```python
from build123d import *

# Parameters (mm, degrees)
F0_W     = 30.4
F0_H     = 20.2
F1_DEPTH = 16
F0_W_2   = 32.4
F0_H_2   = 22.4
F2_DEPTH = 16
F3_DEPTH = 15
F4_R     = 0.25
F5_R     = 0.25
F6_R     = 0.6


with BuildPart() as f1:
    # F0 (on Top) → F1 (new body)
    with BuildSketch(Plane.XY):
        Rectangle(F0_W, F0_H)
    extrude(amount=-F1_DEPTH)

    # F0 (on Top) → F2 (join)
    with BuildSketch(Plane.XY):
        Rectangle(F0_W_2, F0_H_2)
        Rectangle(F0_W, F0_H, mode=Mode.SUBTRACT)
    extrude(amount=-F2_DEPTH)

    # F0 (on Top) → F3 (join)
    with BuildSketch(Plane.XY):
        Rectangle(F0_W_2, F0_H_2)
        Rectangle(F0_W, F0_H, mode=Mode.SUBTRACT)
    extrude(amount=F3_DEPTH)

    # F4
    f4_edges = [f1.edges().sort_by_distance(p)[0] for p in [
        (-15.2, 0, 15),
    ]]
    fillet(f4_edges, radius=F4_R)

    # F5
    f5_edges = [f1.edges().sort_by_distance(p)[0] for p in [
        (0, 10.1, 15),
        (15.2, 0, 15),
        (0, -10.1, 15),
    ]]
    fillet(f5_edges, radius=F5_R)

    # F6
    f6_edges = [f1.edges().sort_by_distance(p)[0] for p in [
        (0, -11.2, 15),
        (-16.2, 0, 15),
        (0, 11.2, 15),
        (16.2, 0, 15),
        (-16.2, -11.2, -0.5),
        (16.2, -11.2, -0.5),
        (16.2, 11.2, -0.5),
        (-16.2, 11.2, -0.5),
        (0, -11.2, -16),
        (16.2, 0, -16),
        (0, 11.2, -16),
        (-16.2, 0, -16),
    ]]
    fillet(f6_edges, radius=F6_R)


solid = f1.part
```
Could you check a few things on this model? Use its own coordinates, in mm. A direction names the side the tool comes from. Coordinates: 2 decimals unless noted, no trailing zeros. Write each loop counter-clockwise with the first axis right and the second up, starting at its lowest first coordinate (ties: lowest second). Pieces come first, ordered by that corner, then holes. Notation, with made-up numbers: (32, 12.25) -> (53, 12.25) arc R25 cw to (53, 27.25) -> close; hole circle Ø8 at (4, -35.5). An arc over 180 degrees is marked (long way). Return JSON: item names as keys, results as strings.
(1) We'd pull the mould along Y, two halves only. Please class faces 3 (the flat face through (0, 0, 0)), 4 (the flat face through (15.2, 0, 7)), 5 (the flat face through (0, -11.2, -1)), 6 (the flat face through (0, 11.2, -1)): +Y half, -Y half, draft (parallel to the pull), parting line (faces both ways), or undercut.
Numbers:
{"face 3": "undercut", "face 4": "undercut", "face 5": "-Y half", "face 6": "+Y half"}
(2) Imagine slicing it at A-A, the plane z = 9.5. Please give me the cut outline in (x, y), then the cut area to 3 significant figures.
Numbers:
{"outline": "(-16.2, -10.6) arc R0.6 ccw to (-15.6, -11.2) -> (15.6, -11.2) arc R0.6 ccw to (16.2, -10.6) -> (16.2, 10.6) arc R0.6 ccw to (15.6, 11.2) -> (-15.6, 11.2) arc R0.6 ccw to (-16.2, 10.6) -> close; hole (-15.2, -10.1) -> (15.2, -10.1) -> (15.2, 10.1) -> (-15.2, 10.1) -> close", "area": "111 mm2"}
(3) I need wall thicknesses on L1, parallel to Y at x = -14, z = 7; L2, parallel to X at y = 4.25, z = 2; L3, parallel to Z at x = 10.5, y = -4. Which ranges of each line are inside material? Lowest first, please.
Numbers:
{"L1": "y = -11.2 to -10.1, 10.1 to 11.2", "L2": "x = -16.2 to -15.2, 15.2 to 16.2", "L3": "z = -16 to 0"}
(4) Imagine slicing it at C-C, the plane x = -5.5. Please give me the cut outline in (y, z).
Numbers:
{"outline": "(-11.2, -15.4) arc R0.6 ccw to (-10.6, -16) -> (10.6, -16) arc R0.6 ccw to (11.2, -15.4) -> (11.2, 14.4) arc R0.6 ccw to (10.6, 15) -> (10.35, 15) arc R0.25 ccw to (10.1, 14.75) -> (10.1, 0) -> (-10.1, 0) -> (-10.1, 14.75) arc R0.25 ccw to (-10.35, 15) -> (-10.6, 15) arc R0.6 ccw to (-11.2, 14.4) -> close"}
(5) Imagine slicing it at B-B, the plane y = 0. Please give me the cut outline in (x, z).
Numbers:
{"outline": "(-16.2, -15.4) arc R0.6 ccw to (-15.6, -16) -> (15.6, -16) arc R0.6 ccw to (16.2, -15.4) -> (16.2, 14.4) arc R0.6 ccw to (15.6, 15) -> (15.45, 15) arc R0.25 ccw to (15.2, 14.75) -> (15.2, 0) -> (-15.2, 0) -> (-15.2, 14.75) arc R0.25 ccw to (-15.45, 15) -> (-15.6, 15) arc R0.6 ccw to (-16.2, 14.4) -> close"}
(6) Which directions (+Z, -Z, +X, -X, +Y, -Y) give clear straight access to the entire face, cutting with the end or side of a thin tool? Please do faces 1 (the flat face through (0, 10.1, 7)), 2 (the flat face through (0, 0, -16)).
Numbers:
{"face 1": "+Z", "face 2": "-Z, +X, -X, +Y, -Y"}
(7) I'm going to push a flat-ended pin straight in: pin 1 (3 mm diameter, centred on x = -8, y = 3.5, fed in from +Z). Where does the tip first touch, or does it pass through?
Numbers:
{"pin 1": "stops at z = 0"}
